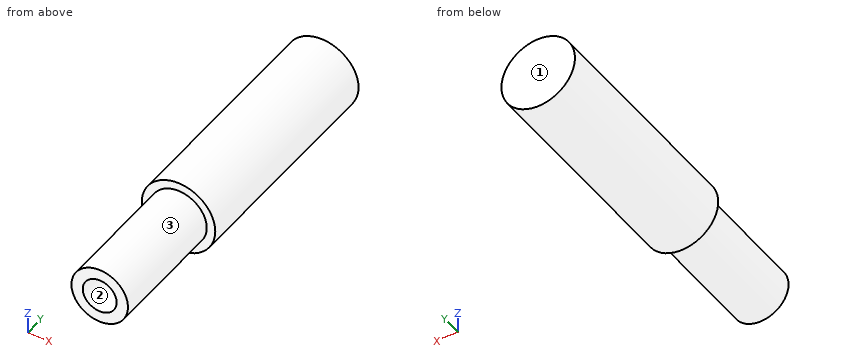
Autodesk Inventor part; units mm, degrees
ref_plane "YZ Plane" through (0, 0, 0) normal (1, 0, 0) x (0, 1, 0)
ref_plane "XZ Plane" through (0, 0, 0) normal (0, 1, 0) x (-1, 0, 0)
ref_plane "XY Plane" through (0, 0, 0) normal (0, 0, 1) x (1, 0, 0)
sketch "スケッチ1" plane through (0, 0, 0) normal (0, 1, 0) x (-1, 0, 0)
  circle A0 centre (0, 0) radius 5
  dimension "d0" = 10
extrude "押し出し1" add sketch "スケッチ1" along normal blind 22
sketch "スケッチ2" plane through (0, 22, 0) normal (0, 1, 0) x (1, 0, 0)
  circle A0 centre (0, 0) radius 6.5
  dimension "d3" = 13
extrude "押し出し2" add sketch "スケッチ2" along normal blind 40
sketch "スケッチ3" plane through (0, 62, 0) normal (0, 1, 0) x (1, 0, 0)
  point P0 (0, 0)
sketch "スケッチ4" plane through (0, 0, 0) normal (0, -1, 0) x (1, 0, 0)
  circle A0 centre (0, 0) radius 3
  dimension "d6" = 6
extrude "押し出し3" cut sketch "スケッチ4" against normal blind 12
properties part number "shaft-k-ki"
Part model, mm, in its own coordinate system. Face numbers are marked on the shaded views. Round coordinates to 2 decimals unless told otherwise and drop trailing zeros. Order: outer loops, then holes, each group sorted by start corner. A loop starts at its lowest first (then second) coordinate and runs counter-clockwise, first axis right, second up. Notation, with made-up numbers: M -33,38 L 7,38 A21 cw 7,67 Z; hole C -25,62 d1. An arc over 180 degrees is marked long. Answer in a Markdown table with one row per item. Add a question column.
Q1. Cut at C-C on z = 0. Give the cut face in (x, y).
Q2. Pin check, flat tip, straight feed: pin 1 (1.5 mm diameter, centred on y = 42.5, z = -2, fed in from +X). Stop position of the tip, or through.
Q3. Cut at A-A on x = 0. Give the cut face in (y, z), and give its area (3 significant figures).
Q4. Wall check: L1, parallel to Z at x = 0, y = 7; L2, parallel to Y at x = 0, z = 1.5; L3, parallel to Y at x = -2, z = 5. Give the ranges that are in metal, low to high. Write a range as from..to.
Q5. Mould opens along X. For the marked faces 1, 2 and 3 say: +X half, -X half, draft (parallel to the pull), parting line (faces both ways), or undercut.
Q6. Cut at B-B on y = 6.5. Give the cut face in (x, z).
Q7. Cut at D-D on y = 49. Give the cut face in (x, z), and give its area (3 significant figures).
Established:
| question | item | result |
|---|---|---|
| 1 | outline | M -6.5,22 L -5,22 L -5,0 L -3,0 L -3,12 L 3,12 L 3,0 L 5,0 L 5,22 L 6.5,22 L 6.5,62 L -6.5,62 Z |
| 2 | pin 1 | stops at x = 6.38 |
| 3 | outline | M 0,-5 L 22,-5 L 22,-6.5 L 62,-6.5 L 62,6.5 L 22,6.5 L 22,5 L 0,5 L 0,3 L 12,3 L 12,-3 L 0,-3 Z |
| 3 | area | 668 mm2 |
| 4 | L1 | z = -5..-3, 3..5 |
| 4 | L2 | y = 12..62 |
| 4 | L3 | y = 22..62 |
| 5 | face 1 | draft |
| 5 | face 2 | undercut |
| 5 | face 3 | parting line |
| 6 | outline | C 0,0 d10; hole C 0,0 d6 |
| 7 | outline | C 0,0 d13 |
| 7 | area | 133 mm2 |
